The listing builds one solid part. Answer for the finished solid, in the listing's coordinates (mm). A direction names the side the tool comes from. Coordinates: 2 decimals unless noted, no trailing zeros. Write each loop counter-clockwise with the first axis right and the second up, starting at its lowest first coordinate (ties: lowest second). Pieces come first, ordered by that corner, then holes.
from build123d import *

# Parameters (mm, degrees)
F0_W     = 20.5790107138
F0_H     = 20.4056631774
F0_W_2   = 13
F0_H_2   = 13.5
F0_R     = 4.75
F1_DEPTH = 5
F2_DEPTH = 1.5


with BuildPart() as f1:
    # F0 (on Top) → F1 (new body)
    with BuildSketch(Plane.XY):
        Rectangle(F0_W, F0_H)
        Rectangle(F0_W_2, F0_H_2, mode=Mode.SUBTRACT)
        Rectangle(F0_W_2, F0_H_2)
        Circle(F0_R, mode=Mode.SUBTRACT)
    extrude(amount=F1_DEPTH)

    # F0 (on Top) → F2 (cut)
    with BuildSketch(Plane.XY):
        Rectangle(F0_W_2, F0_H_2)
        Circle(F0_R, mode=Mode.SUBTRACT)
    extrude(amount=F2_DEPTH, mode=Mode.SUBTRACT)


solid = f1.part
1. Section C-C on z = 0.75 is taken. Give the vertices of the cut face in (x, y).
Results found:
outline: (-10.29, -10.2) - (10.29, -10.2) - (10.29, 10.2) - (-10.29, 10.2) - close; hole (-6.5, -6.75) - (6.5, -6.75) - (6.5, 6.75) - (-6.5, 6.75) - close
2. Section A-A on x = 0 is taken. Give the vertices of the cut face in (y, z).
Results found:
outline: (-10.2, 0) - (-6.75, 0) - (-6.75, 1.5) - (-4.75, 1.5) - (-4.75, 5) - (-10.2, 5) - close; (4.75, 1.5) - (6.75, 1.5) - (6.75, 0) - (10.2, 0) - (10.2, 5) - (4.75, 5) - close
3. Section D-D on y = 5 is taken. Give the vertices of the cut face in (x, z).
Results found:
outline: (-10.29, 0) - (-6.5, 0) - (-6.5, 1.5) - (6.5, 1.5) - (6.5, 0) - (10.29, 0) - (10.29, 5) - (-10.29, 5) - close
4. For a pull along Y with two mould halves and no side action, classify faces 3 (the flat face through (6.5, 0, 1)), 4 (the flat face through (0, -10.203, 2)), 5 (the flat face through (-10.29, 0, 2)) as pulls with the +Y half, pulls with the -Y half, needs draft (parallel to the pull), parting line crosses it, or undercut.
Results found:
face 3: undercut
face 4: pulls with the -Y half
face 5: needs draft
5. Flat-ended cylindrical pins translate along their axes: P1, Ø4, axis at x = -0.5, y = -1, coming from the -Z side; P2, Ø1.5, axis at x = 5, y = -3, coming from the -Z side. Find the tip coordinate at first contact, or state that the pin passes through.
Results found:
P1: passes through
P2: stops at z = 1.5
6. Find the intervals of material crossed by L1, parallel to Y at x = -5.25, z = 1.1; L2, parallel to Y at x = 0, z = 2.3; L3, parallel to X at y = -5.25, z = 0.9, in increasing order.
Results found:
L1: y = -10.2 to -6.75, 6.75 to 10.2
L2: y = -10.2 to -4.75, 4.75 to 10.2
L3: x = -10.29 to -6.5, 6.5 to 10.29
7. A tool of negligible diameter and unlimited length cuts with its end or side. For faces 1 (the flat face through (0, -6.75, 1)), 2 (the cylindrical face through (2.192, -4.214, 3.226)), from which of +Z, -Z, +X, -X, +Y, -Y can it reach the whole face along a straight path? Write none if from no direction.
Results found:
face 1: -Z
face 2: +Z, -Z
8. Section B-B on y = 0 is taken. Give the vertices of the cut face in (x, z), then the cut area to 3 significant figures.
Results found:
outline: (-10.29, 0) - (-6.5, 0) - (-6.5, 1.5) - (-4.75, 1.5) - (-4.75, 5) - (-10.29, 5) - close; (4.75, 1.5) - (6.5, 1.5) - (6.5, 0) - (10.29, 0) - (10.29, 5) - (4.75, 5) - close
area: 50.1 mm2
